```python
from build123d import *

# Parameters (mm, degrees)
FILLET1_R          = 10
SKETCH6_R          = 1.15
CUT_EXTRUDE1_DEPTH = 10


with BuildPart() as part:
    # Sketch2 → Revolve1 (revolve)
    with BuildSketch(Plane.XY, mode=Mode.PRIVATE) as revolve1_sk:
        Polygon((0, 4), (-3.05, 4), (-3.05, 3), (-3.05, 0), (-5.05, 0), (-5.05, 4), (-28.5, 4), (-28.5, 0), (-30.5, 0), (-30.5, 4), (-30.5, 6), (0, 6), align=None)
    revolve(revolve1_sk.sketch.rotate(Axis((0, 0, 0), (0, 1, 0)), 270), axis=Axis((0, 0, 0), (0, 1, 0)))

    # Fillet1
    # the kernel refuses this fillet: 10 mm, written as the material it adds along each edge
    with BuildSketch(Plane(origin=(0, 4, 0), x_dir=(0, 0, -1), z_dir=(1, 0, 0))) as fillet1_piece_1:
        with BuildLine():
            CenterArc((20.5, -10), FILLET1_R, 36.869897646, 53.130102354)
            Line((28.5, -4), (28.66, -3.88))
            ThreePointArc((28.66, -3.88), (28.7, -2), (28.7, 0))
            Line((28.7, 0), (28.5, 0.2))
            Line((28.5, 0.2), (20.5, 0.2))
            Line((20.5, 0.2), (20.5, 0))
        make_face()
    revolve(axis=Axis((0, 4, 0), (0, 1, 0)))
    with BuildSketch(Plane(origin=(0, 4, 0), x_dir=(0, 0, -1), z_dir=(1, 0, 0))) as fillet1_piece_2:
        with BuildLine():
            CenterArc((13.05, -10), FILLET1_R, 90, 53.130102354)
            Line((13.05, 0), (13.05, 0.2))
            Line((13.05, 0.2), (5.05, 0.2))
            Line((5.05, 0.2), (4.85, 0))
            ThreePointArc((4.85, 0), (4.85, -2), (4.89, -3.88))
            Line((4.89, -3.88), (5.05, -4))
        make_face()
    revolve(axis=Axis((0, 4, 0), (0, 1, 0)))

    # Sketch6 → Cut-Extrude1 (cut)
    with BuildSketch(Plane(origin=(0, 6, 0), x_dir=(1, 0, 0), z_dir=(0, 1, 0))):
        with Locations(Location((-11.275, 16.4, 0), (0, 0, 270))):
            Circle(SKETCH6_R)
        with Locations(Location((-11.275, -16.4, 0), (0, 0, 270))):
            Circle(SKETCH6_R)
    extrude(amount=-CUT_EXTRUDE1_DEPTH, mode=Mode.SUBTRACT)


solid = part.part
```
Check sheet for the modelled part. Datum: model origin and axes. Units: mm. A direction names the side the tool comes from. Round coordinates to 2 decimals unless told otherwise and drop trailing zeros. Order: outer loops, then holes, each group sorted by start corner. A loop starts at its lowest first (then second) coordinate and runs counter-clockwise, first axis right, second up. Notation, with made-up numbers: (-2.75, -22) - (3.25, -22) arc R24 ccw to (3.25, 0) - close; hole circle Ø10 at (26, 87.25). An arc over 180 degrees is marked (long way). Write item = value, one per line.
Q1. Go/stop test with flat-tipped pins: pin 1 (10 mm diameter, centred on x = 8.5, z = -14.5, fed in from -Y); pin 2 (3 mm diameter, centred on x = 0.5, z = 0, fed in from -Y); pin 3 (2.5 mm diameter, centred on x = -11.275, z = -16.4, fed in from +Y); pin 4 (1.5 mm diameter, centred on y = 3.5, z = 4, fed in from +X). Record where each tip stops, or that it passes through.
Computed:
pin_1 = 3.91
pin_2 = 4
pin_3 = 6
pin_4 = 30.33
Q2. Draft check along X on faces 1 (the face through (29.775, 2.958, 6.612)), 2 (the face through (3.3, 0, -0.1)), 3 (the face through (-10.5, 5.01, -17.25)). Enter one of: pulls with the +X half, pulls with the -X half, needs draft (parallel to the pull), parting line crosses it, or undercut.
Computed:
face_1 = parting line crosses it
face_2 = needs draft
face_3 = undercut
Q3. Section check B-B (z = 0). Record the boundary of the cut face in (x, y), and give its area (3 significant figures).
Computed:
outline = (-30.5, 0) - (-28.5, 0) arc R10 cw to (-20.5, 4) - (-13.05, 4) arc R10 cw to (-5.05, 0) - (-3.05, 0) - (-3.05, 4) - (3.05, 4) - (3.05, 0) - (5.05, 0) arc R10 cw to (13.05, 4) - (20.5, 4) arc R10 cw to (28.5, 0) - (30.5, 0) - (30.5, 6) - (-30.5, 6) - close
area = 193 mm^2
Q4. Thickness scan on line 1 along Z through (x, y) = (-2, 2.5); line 2 along Z through (x, y) = (-4, 0.5); line 3 along X through (y, z) = (2, -3.5). Record the ranges inside material, lowest first.
Computed:
line_1 = -30.43 to -25.69, -7.52 to -2.3, 2.3 to 7.52, 25.69 to 30.43
line_2 = -30.24 to -27.81, -3.7 to 3.7, 27.81 to 30.24
line_3 = -30.3 to -26.27, -6.12 to 6.12, 26.27 to 30.3
Q5. Tool access check on faces 4 (the face through (1.856, 2.028, 2.42)), 5 (the face through (-14, 0, -25)). Record the directions out of +Z, -Z, +X, -X, +Y, -Y that give a thin tool (end or side, any length) a straight path to the whole face; none if there is none.
Computed:
face_4 = -Y
face_5 = +Z, -Z, +X, -X, -Y
Q6. Section check C-C (y = 3.25). Record the boundary of the cut face in (x, z).
Computed:
outline = circle Ø61 at (0, 0); circle Ø18.5 at (0, 0); hole circle Ø48.6 at (0, 0); hole circle Ø6.1 at (0, 0)
Q7. Section check A-A (x = 0). Record the boundary of the cut face in (y, z), and give its area (3 significant figures).
Computed:
outline = (0, -30.5) - (6, -30.5) - (6, 30.5) - (0, 30.5) - (0, 28.5) arc R10 cw to (4, 20.5) - (4, 13.05) arc R10 cw to (0, 5.05) - (0, 3.05) - (4, 3.05) - (4, -3.05) - (0, -3.05) - (0, -5.05) arc R10 cw to (4, -13.05) - (4, -20.5) arc R10 cw to (0, -28.5) - close
area = 193 mm^2
